Geometry: see drawing. Coordinates: mm, zero at the bounding-box minimum. Coordinates: 2 decimals unless noted, no trailing zeros. Order: outer loops, then holes, each group sorted by start corner. A loop starts at its lowest first (then second) coordinate and runs counter-clockwise, first axis right, second up.
Item 1: Contact query for flat-ended pins moving along their axis: P1, Ø1.6, axis at y = 114.5, z = 1.5, coming from the +X side (3 decimals); P2, Ø1, axis at x = 113.5, z = 1.5, coming from the -Y side; P3, Ø1.6, axis at y = 60.5, z = 1, coming from the -X side (3 decimals). Output: stop coordinate, or through.
Item 2: Section B-B on x = 115. Return the cut outline in (y, z) (3 decimals).
Item 3: Ray query, line 1 (X direction, y = 15, z = 1); line 2 (Y direction, x = 17.5, z = 0.85) (3 decimals); line 3 (X direction, y = 9.5, z = 1.9). Return the intervals inside material, ascending.
Item 4: Section C-C on y = 59. Return the cut outline in (x, z) (3 decimals).
Item 5: Section A-A on y = 37.5. Return the cut outline in (x, z) (3 decimals), then the cut area to 3 significant figures.
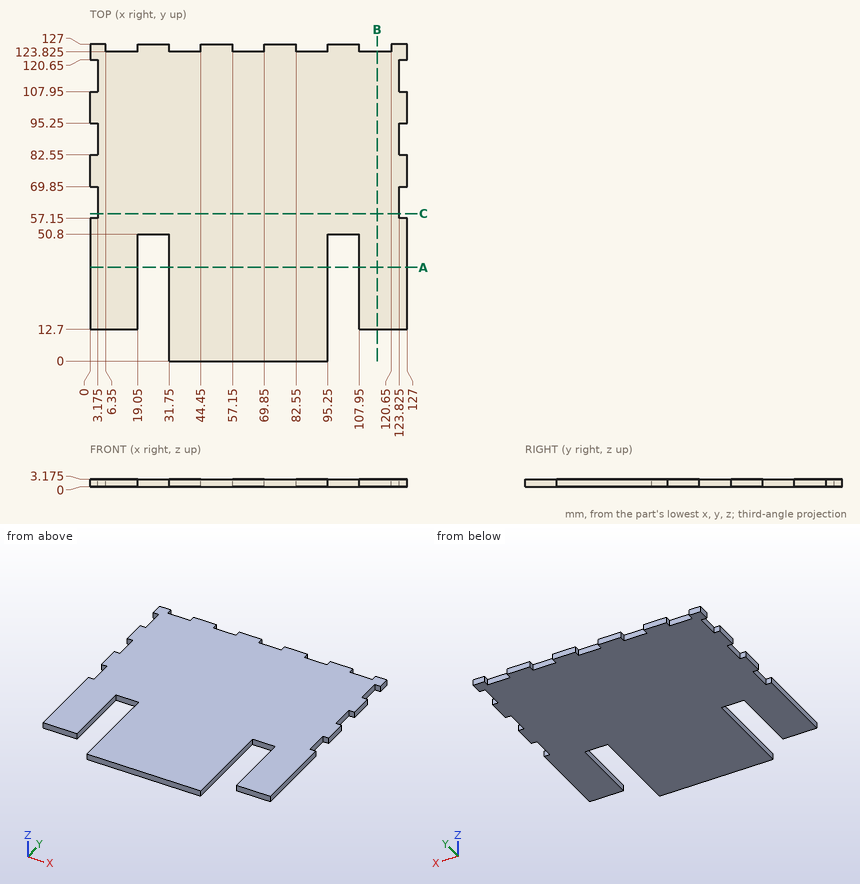
Answer list:
1. P1: stops at x = 123.825
1. P2: stops at y = 12.7
1. P3: stops at x = 3.175
2. outline: (12.7, 0) - (123.825, 0) - (123.825, 3.175) - (12.7, 3.175) - close
3. line 1: x = 0 to 19.05, 31.75 to 95.25, 107.95 to 127
3. line 2: y = 12.7 to 123.825
3. line 3: x = 31.75 to 95.25
4. outline: (3.175, 0) - (123.825, 0) - (123.825, 3.175) - (3.175, 3.175) - close
5. outline: (0, 0) - (19.05, 0) - (19.05, 3.175) - (0, 3.175) - close; (31.75, 0) - (95.25, 0) - (95.25, 3.175) - (31.75, 3.175) - close; (107.95, 0) - (127, 0) - (127, 3.175) - (107.95, 3.175) - close
5. area: 323 mm2
